Build history of the part. All positions in model axes, mm. A direction names the side the tool comes from. Give positions to 0.01 mm unless a question says otherwise; leave off trailing zeros. Loops run counter-clockwise (first coordinate to the right, second up) from the corner with the lowest first, then second, coordinate; pieces in that order, holes last.
1) Band-saw the part on C-C on x = -30.4. List the corners of the cut face in (y, z).
2) Band-saw the part on A-A on y = -30. List the corners of the cut face in (x, z), then the cut area to 3 significant figures.
3) Flat gauge pins, fed straight in: P1, Ø5.5, axis at y = -15, z = 75, coming from the -X side; P2, Ø4.5, axis at x = 30.4, z = 17.4, coming from the +Y side; P3, Ø1, axis at x = -21.5, y = -3.5, coming from the -Z side; P4, Ø20, axis at y = -11, z = 54, coming from the +X side. Where does each tip first touch, or does it go through?
4) Band-saw the part on D-D on x = -4.5. List the corners of the cut face in (y, z).
5) Band-saw the part on B-B on z = 75. List the corners of the cut face in (x, y), then the cut area to 3 significant figures.
6) 3-axis set-ups, long thin cutter, end or side, ignore diameter. For faces 1 (the flat face through (-31, -5, 37)), 2 (the flat face through (-58, 0, 70)), 3 (the flat face through (1, 5, 61)), 4 (the flat face through (37.5, -4.5, 45.3)), 5 (the flat face through (0, -28.4, 62)): which of +Z, -Z, +X, -X, +Y, -Y reach the whole face in a straight line?
7) Two-plate mould, pull along Z, no slides. Class faces 6 (the flat face through (-31, 0, 12.4)), 7 (the cylindrical face through (29.34, -0.07, 51.91)), 8 (the flat face through (70, 0, 75)): +Z half, -Z half, draft (parallel to the pull), parting line (faces both ways), or undercut.
8) Wall check: line 1 (Y direction, x = -67, z = 75); line 2 (Z direction, x = -30.4, y = -1); line 3 (X direction, y = 0, z = 53.5). Give the ranges that are in metal, low to high.
```python
from build123d import *

# Parameters (mm, degrees)
SKETCH_1_W               = 140
SKETCH_1_H               = 10
EXTRUDE_1_DEPTH          = 80
SKETCH_2_W               = 32.5
SKETCH_2_H               = 70
CUT_EXTRUDE_1_DEPTH      = 107.77078252
SKETCH_4_W               = 55
SKETCH_4_H               = 10
CUT_EXTRUDE_2_DEPTH      = 60
SKETCH_5_W               = 8
SKETCH_5_H               = 40
EXTRUDE_2_DEPTH          = 10
CUT_EXTRUDE_START        = -12.4
SKETCH_6_W               = 10
SKETCH_6_H               = 10
CUT_EXTRUDE_3_DEPTH      = 12.4
SKETCH_7_W               = 75
SKETCH_7_H               = 4
EXTRUDE_3_DEPTH          = 30
CUT_EXTRUDE_4_DEPTH      = 27
CUT_EXTRUDE_5_DEPTH      = 159.268758762
CUT_EXTRUDE_5_DEPTH_BACK = 159.268758762
SKETCH_9_R               = 1.75
CUT_EXTRUDE_6_DEPTH      = 114.578166916
CUT_EXTRUDE_6_DEPTH_BACK = 114.578166916
SKETCH_10_R              = 1.75
SKETCH_11_W              = 47.6
SKETCH_11_H              = 10
EXTRUDE_4_DEPTH          = 3
SKETCH_12_W              = 47.6
SKETCH_12_H              = 10
EXTRUDE_5_DEPTH          = 3


with BuildPart() as part:
    # 草图1 → 凸台-拉伸1 (new body)
    with BuildSketch(Plane.XY):
        Rectangle(SKETCH_1_W, SKETCH_1_H)
    extrude(amount=EXTRUDE_1_DEPTH)

    # 草图2 → 切除-拉伸1 (cut, through all)
    with BuildSketch(Plane(origin=(0, 5, 0), x_dir=(1, 0, 0), z_dir=(0, 1, 0))):
        with Locations((-53.75, -35)):
            Rectangle(SKETCH_2_W, SKETCH_2_H)
        with Locations((53.75, -35)):
            Rectangle(SKETCH_2_W, SKETCH_2_H)
    extrude(amount=-CUT_EXTRUDE_1_DEPTH, mode=Mode.SUBTRACT)

    # 草图4 → 切除-拉伸2 (cut)
    with BuildSketch(Plane(origin=(0, 0, 0), x_dir=(-1, 0, 0), z_dir=(0, 0, -1))):
        Rectangle(SKETCH_4_W, SKETCH_4_H)
    extrude(amount=-CUT_EXTRUDE_2_DEPTH, mode=Mode.SUBTRACT)

    # 草图5 → 凸台-拉伸2 (add)
    with BuildSketch(Plane(origin=(0, 0, 70), x_dir=(-1, 0, 0), z_dir=(0, 0, -1))):
        with Locations((-66, 0)):
            Rectangle(SKETCH_5_W, SKETCH_5_H)
        with Locations((66, 0)):
            Rectangle(SKETCH_5_W, SKETCH_5_H)
    extrude(amount=-EXTRUDE_2_DEPTH)

    # 草图6 → 切除-拉伸3 (cut)
    with BuildSketch(Plane(origin=(0, 0, 0), x_dir=(-1, 0, 0), z_dir=(0, 0, -1)).offset(CUT_EXTRUDE_START)):
        with Locations((32.5, 0)):
            Rectangle(SKETCH_6_W, SKETCH_6_H)
        with Locations((-32.5, 0)):
            Rectangle(SKETCH_6_W, SKETCH_6_H)
    extrude(amount=CUT_EXTRUDE_3_DEPTH, mode=Mode.SUBTRACT)

    # 草图7 → 凸台-拉伸3 (add)
    with BuildSketch(Plane.XZ.offset(5)):
        with Locations((0, 62)):
            Rectangle(SKETCH_7_W, SKETCH_7_H)
    extrude(amount=EXTRUDE_3_DEPTH)

    # 草图8 → 切除-拉伸4 (cut)
    with BuildSketch(Plane(origin=(0, 0, 60), x_dir=(-1, 0, 0), z_dir=(0, 0, -1))):
        with BuildLine():
            Line((-33.5, -28.4), (33.5, -28.4))
            ThreePointArc((33.5, -28.4), (35.1, -30), (33.5, -31.6))
            Line((33.5, -31.6), (-33.5, -31.6))
            ThreePointArc((-33.5, -31.6), (-35.1, -30), (-33.5, -28.4))
        make_face()
    extrude(amount=-CUT_EXTRUDE_4_DEPTH, mode=Mode.SUBTRACT)

    # 草图9 → 切除-拉伸5 (cut, two sides: drawn at the far end of the back side and taken through both)
    with BuildSketch(Plane(origin=(-62, 0, 0), x_dir=(0, 0, -1), z_dir=(1, 0, 0)).offset(-CUT_EXTRUDE_5_DEPTH_BACK)):
        with Locations((-75, 15)):
            Circle(SKETCH_9_R)
        with Locations((-75, -15)):
            Circle(SKETCH_9_R)
    extrude(amount=CUT_EXTRUDE_5_DEPTH + CUT_EXTRUDE_5_DEPTH_BACK, mode=Mode.SUBTRACT)

    # 草图10 → 切除-拉伸6 (cut, two sides: drawn at the far end of the back side and taken through both)
    with BuildSketch(Plane(origin=(0, 5, 0), x_dir=(1, 0, 0), z_dir=(0, 1, 0)).offset(-CUT_EXTRUDE_6_DEPTH_BACK)):
        with Locations(Location((30.4, -53.3, 0), (0, 0, 270))):
            Circle(SKETCH_10_R)
        with Locations(Location((30.4, -17.4, 0), (0, 0, 270))):
            Circle(SKETCH_10_R)
        with Locations(Location((-30.4, -17.4, 0), (0, 0, 270))):
            Circle(SKETCH_10_R)
        with Locations(Location((-30.4, -53.3, 0), (0, 0, 270))):
            Circle(SKETCH_10_R)
    extrude(amount=CUT_EXTRUDE_6_DEPTH + CUT_EXTRUDE_6_DEPTH_BACK, mode=Mode.SUBTRACT)

    # 草图11 → 凸台-拉伸4 (add)
    with BuildSketch(Plane.ZY.offset(-27.5)):
        with Locations((36.2, 0)):
            Rectangle(SKETCH_11_W, SKETCH_11_H)
    extrude(amount=EXTRUDE_4_DEPTH)

    # 草图12 → 凸台-拉伸5 (add)
    with BuildSketch(Plane(origin=(-27.5, 0, 0), x_dir=(0, 0, -1), z_dir=(1, 0, 0))):
        with Locations((-36.2, 0)):
            Rectangle(SKETCH_12_W, SKETCH_12_H)
    extrude(amount=EXTRUDE_5_DEPTH)


solid = part.part
```
Findings below:
1. outline: (-35, 60) - (-31.6, 60) - (-31.6, 64) - (-35, 64) - close; (-28.4, 60) - (-5, 60) - (-5, 55.05) - (5, 55.05) - (5, 80) - (-5, 80) - (-5, 64) - (-28.4, 64) - close; (-5, 12.4) - (5, 12.4) - (5, 15.65) - (-5, 15.65) - close; (-5, 19.15) - (5, 19.15) - (5, 51.55) - (-5, 51.55) - close
2. outline: (-37.5, 60) - (-35.1, 60) - (-35.1, 64) - (-37.5, 64) - close; (35.1, 60) - (37.5, 60) - (37.5, 64) - (35.1, 64) - close
2. area: 19.2 mm2
3. P1: stops at x = -70
3. P2: stops at y = 5
3. P3: stops at z = 60
3. P4: stops at x = 37.5
4. outline: (-35, 60) - (-31.6, 60) - (-31.6, 64) - (-35, 64) - close; (-28.4, 60) - (5, 60) - (5, 80) - (-5, 80) - (-5, 64) - (-28.4, 64) - close
5. outline: (-70, -20) - (-62, -20) - (-62, -16.75) - (-70, -16.75) - close; (-70, -13.25) - (-62, -13.25) - (-62, -5) - (62, -5) - (62, -13.25) - (70, -13.25) - (70, 13.25) - (62, 13.25) - (62, 5) - (-62, 5) - (-62, 13.25) - (-70, 13.25) - close; (-70, 16.75) - (-62, 16.75) - (-62, 20) - (-70, 20) - close; (62, -20) - (70, -20) - (70, -16.75) - (62, -16.75) - close; (62, 16.75) - (70, 16.75) - (70, 20) - (62, 20) - close
5. area: 1,770 mm2
6. face 1: -Z, +X, -X, -Y
6. face 2: -Z, -X, +Y, -Y
6. face 3: +Z, -Z, +Y
6. face 4: -Z, +X, +Y, -Y
6. face 5: +Z, -Z
7. face 6: -Z half
7. face 7: undercut
7. face 8: draft
8. line 1: y = -20 to -16.75, -13.25 to 13.25, 16.75 to 20
8. line 2: z = 12.4 to 15.65, 19.15 to 51.55, 55.05 to 80
8. line 3: x = -37.5 to -32.14, -28.66 to -24.5, 24.5 to 28.66, 32.14 to 37.5
